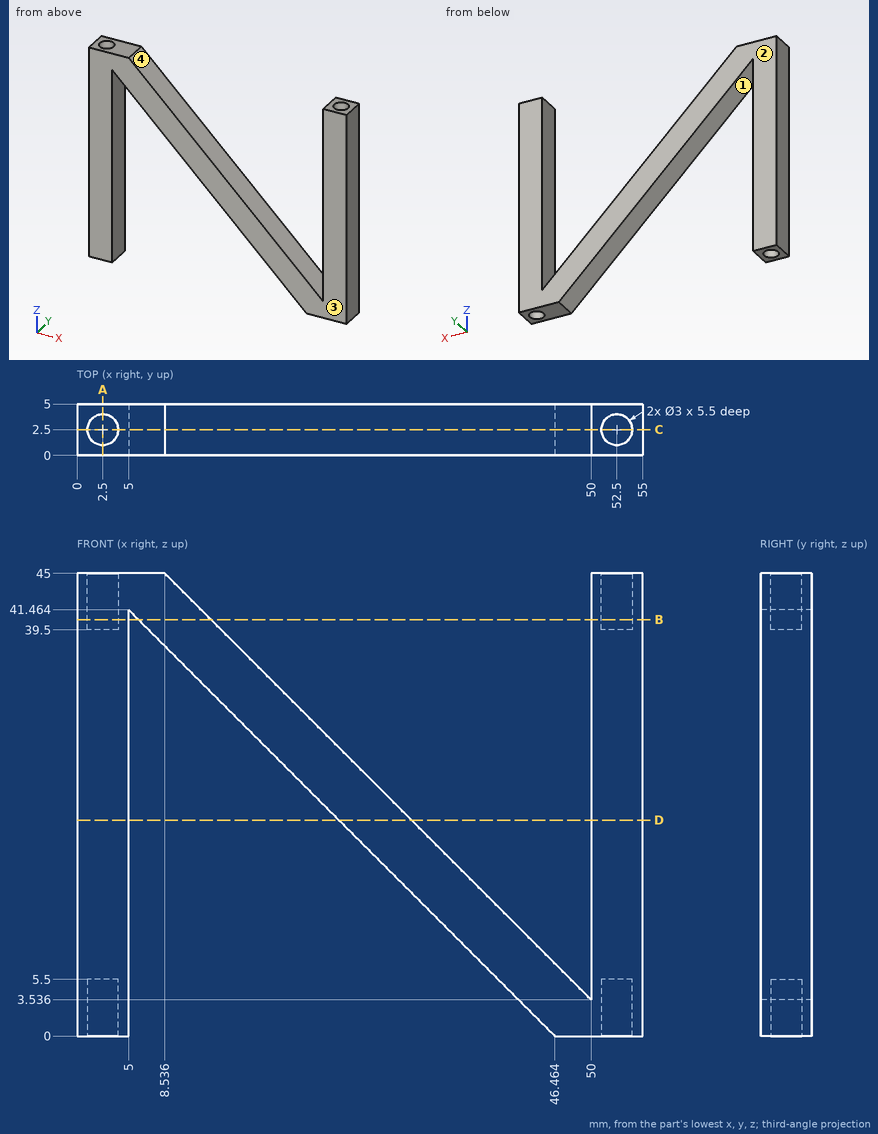
The drawing under review shows one solid part. Ordinate dimensions are in mm from its lowest x, y, z. A direction names the side the tool comes from. Round coordinates to 2 decimals unless told otherwise and drop trailing zeros. Write each loop counter-clockwise with the first axis right and the second up, starting at its lowest first coordinate (ties: lowest second). Pieces come first, ordered by that corner, then holes. Notation, with made-up numbers: (31, -10.5) - (73, -10.5) arc R22 ccw to (73, 24.5) - close; hole circle Ø4 at (-1.5, -37). An arc over 180 degrees is marked (long way). One line per question, with ' | ' between items.
Item 1: Add section A-A, the plane x = 2.5. Give the boundary of the cut face in (y, z), then the cut area to 3 significant figures.
Resolved:
outline: (0, 0) - (1, 0) - (1, 5.5) - (4, 5.5) - (4, 0) - (5, 0) - (5, 45) - (4, 45) - (4, 39.5) - (1, 39.5) - (1, 45) - (0, 45) - close | area: 192 mm2
Item 2: The part is to be moulded in two halves that separate along X. For the marked faces 3 and 4, say which applies: pulls with the +X half, pulls with the -X half, needs draft (parallel to the pull), parting line crosses it, or undercut.
Resolved:
face 3: needs draft | face 4: undercut
Item 3: Add section B-B, the plane z = 40.5. Give the boundary of the cut face in (x, y) (1 decimal).
Resolved:
outline: (0, 0) - (5, 0) - (5, 5) - (0, 5) - close; (6, 0) - (13, 0) - (13, 5) - (6, 5) - close; (50, 0) - (55, 0) - (55, 5) - (50, 5) - close; hole circle Ø3 at (2.5, 2.5); hole circle Ø3 at (52.5, 2.5)
Item 4: For P1, Ø2.5, axis at x = 2.5, y = 2.5, coming from the -Z side; P2, Ø3, axis at x = 40.5, y = 3.5, coming from the -Z side (1 decimal), all flat-tipped, find the tip position at first contact; note any pin that passes through.
Resolved:
P1: stops at z = 5.5 | P2: stops at z = 4.5
Item 5: For the marked faces 1 and 2, list the 3-axis set-ups (+Z, -Z, +X, -X, +Y, -Y) from which the entire face can be reached by the end or side of a thin tool; tool diameter is ignored.
Resolved:
face 1: -Z, +Y, -Y | face 2: +Z, -Z, +X, -X, +Y
Item 6: To check wall thickness, follow probe 1 along Y at (x, z) = (2.5, 1.5); probe 2 along X at (y, z) = (1.1, 7) (1 decimal); probe 3 along X at (y, z) = (2.2, 38) (1 decimal). State the ranges of each line that lie inside material, in increasing order.
Resolved:
probe 1: y = 0 to 1, 4 to 5 | probe 2: x = 0 to 5, 39.5 to 46.5, 50 to 55 | probe 3: x = 0 to 5, 8.5 to 15.5, 50 to 55
Item 7: Add section C-C, the plane y = 2.5. Give the boundary of the cut face in (x, z) (1 decimal).
Resolved:
outline: (0, 0) - (1, 0) - (1, 5.5) - (4, 5.5) - (4, 0) - (5, 0) - (5, 41.5) - (46.5, 0) - (51, 0) - (51, 5.5) - (54, 5.5) - (54, 0) - (55, 0) - (55, 45) - (54, 45) - (54, 39.5) - (51, 39.5) - (51, 45) - (50, 45) - (50, 3.5) - (8.5, 45) - (4, 45) - (4, 39.5) - (1, 39.5) - (1, 45) - (0, 45) - close
Item 8: Add section D-D, the plane z = 21. Give the boundary of the cut face in (x, y) (1 decimal).
Resolved:
outline: (0, 0) - (5, 0) - (5, 5) - (0, 5) - close; (25.5, 0) - (32.5, 0) - (32.5, 5) - (25.5, 5) - close; (50, 0) - (55, 0) - (55, 5) - (50, 5) - close
